Geometry check sheet. Reference: the model listing, model coordinates, mm. Face numbers are marked on the shaded views. A direction names the side the tool comes from. Round coordinates to 2 decimals unless told otherwise and drop trailing zeros. Loops run counter-clockwise (first coordinate to the right, second up) from the corner with the lowest first, then second, coordinate; pieces in that order, holes last. Notation, with made-up numbers: M 29.25,2.25 L 85.25,2.25 A25 cw 85.25,35.25 Z; hole C 2.25,-1.5 d11. An arc over 180 degrees is marked long. Use one line per item in the form item = value. Start each with the question number.
1. Go/stop test with flat-tipped pins: pin 1 (5 mm diameter, centred on x = 35, y = 8.5, fed in from -Z); pin 2 (12 mm diameter, centred on x = 78.5, z = -11, fed in from +Y); pin 3 (1.5 mm diameter, centred on x = 56.5, z = -11, fed in from -Y). Record where each tip stops, or that it passes through.
2. Cross-section at A-A (x = 85). Record the boundary of the cut face in (y, z).
3. Set-up check for the marked faces 1 and 2: record each of +Z, -Z, +X, -X, +Y, -Y from which the full face is reachable in a straight line by a thin tool's end or side.
4. Cross-section at C-C (z = -17.75). Record the boundary of the cut face in (x, y), then the cut area to 3 significant figures.
5. Material ranges on line 1 (Z direction, x = 23.5, y = 10); line 2 (Y direction, x = 7, z = -23.75); line 3 (Y direction, x = 87, z = -10.25), recorded low to high.
6. Cross-section at B-B (y = 7). Record the boundary of the cut face in (x, z), then the cut area to 3 significant figures.
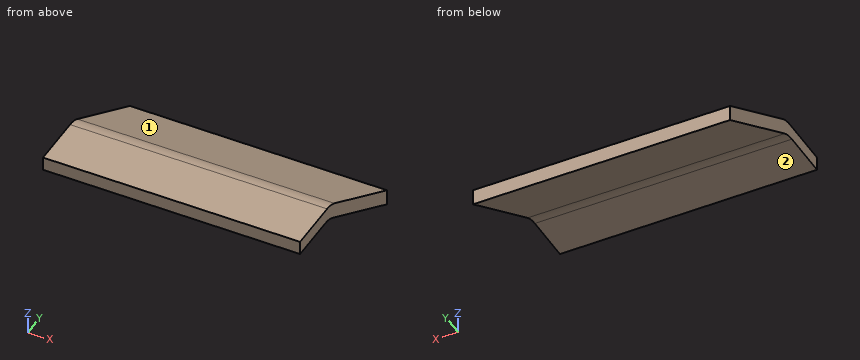
```python
from build123d import *

# Parameters (mm, degrees)
BOSS_EXTRUDE1_DEPTH = 92
FILLET1_R           = 10
FILLET2_R           = 10


with BuildPart() as part:
    # Sketch1 → Boss-Extrude1 (new body)
    with BuildSketch(Plane(origin=(0, 0, 0), x_dir=(0, 0, -1), z_dir=(1, 0, 0))):
        Polygon((0, 0), (0, 21.339745962), (22.320508076, 60), (28.094010768, 60), (5, 20), (5, 0), align=None)
    extrude(amount=BOSS_EXTRUDE1_DEPTH)

    # Fillet1
    fillet1_edges = [part.edges().sort_by_distance(p)[0] for p in [
        (46, 21.339745962, 0),
    ]]
    fillet(fillet1_edges, radius=FILLET1_R)

    # Fillet2
    fillet2_edges = [part.edges().sort_by_distance(p)[0] for p in [
        (46, 20, -5),
    ]]
    fillet(fillet2_edges, radius=FILLET2_R)


solid = part.part
```
Reported:
q1.pin_1 = -5
q1.pin_2 = 50.78
q1.pin_3 = 29.09
q2.outline = M 0,-5 L 17.32,-5 A10 cw 22.32,-6.34 L 60,-28.09 L 60,-22.32 L 23.66,-1.34 A10 ccw 18.66,0 L 0,0 Z
q3.face_1 = +Z, +X, -X, +Y
q3.face_2 = -Z, +X, -X, -Y
q4.outline = M 0,42.08 L 92,42.08 L 92,52.08 L 0,52.08 Z
q4.area = 920 mm²
q5.line_1 = -5 to 0
q5.line_2 = 52.48 to 60
q5.line_3 = 29.09 to 39.09
q6.outline = M 0,-5 L 92,-5 L 92,0 L 0,0 Z
q6.area = 460 mm²
